Can you work these out from the model? Positions are in its coordinate system, mm. Face numbers are marked on the shaded views. A direction names the side the tool comes from. Give positions to 0.01 mm unless a question says otherwise; leave off trailing zeros. Order: outer loops, then holes, each group sorted by start corner. A loop starts at its lowest first (then second) coordinate and runs counter-clockwise, first axis right, second up. Notation, with made-up numbers: M 79,16 L 89,16 A31 ccw 89,52 Z; hole C 40.5,-15 d11. An arc over 180 degrees is marked long. Use one line per item in the form item = value. Start each with the question number.
1. We'd pull the mould along X, two halves only. Please class the marked faces 1, 2, 3 and 4: +X half, -X half, draft (parallel to the pull), parting line (faces both ways), or undercut.
2. I want a section at A-A, the plane z = -29.1. List the corners of the cut face in (x, y) for me, and give its area (3 significant figures).
3. I want a section at C-C, the plane z = -41.5. List the corners of the cut face in (x, y) for me.
4. Will this pin go through, and if not, where does the flat tip stop? P1, Ø11.5, axis at y = 397.93, z = -29.1, coming from the -X side.
5. I need wall thicknesses on L1, parallel to Y at x = -13.5, z = -29.1; L2, parallel to Z at x = 6, y = 488; L3, parallel to X at y = 475, z = -33.5. Which ranges of each line are inside material? Lowest first, please.
6. For the marked faces 5 and 6, which set-ups out of +Z, -Z, +X, -X, +Y, -Y let a thin tool reach every point of the face, with its end or its side?
7. I want a section at B-B, the plane x = -3.75. List the corners of the cut face in (y, z) for me, and give its area (3 significant figures).
8. I want a section at D-D, the plane y = 459. List the corners of the cut face in (x, z) for me, and give its area (3 significant figures).
```python
from build123d import *

# Parameters (mm, degrees)
CROQUIS1_W                        = 30
CROQUIS1_H                        = 119.965463257
SALIENTE_EXTRUIR1_DEPTH           = 30
CROQUIS2_W                        = 24
CROQUIS2_H                        = 24
CORTAR_EXTRUIR1_DEPTH             = 120.965463257
DI_METRO_DE_TALADRO_9_0_9_1_D     = 9
DI_METRO_DE_TALADRO_9_0_9_1_DEPTH = 3
DI_METRO_DE_TALADRO_9_0_9_2_D     = 9
DI_METRO_DE_TALADRO_9_0_9_2_DEPTH = 30
REDONDEO1_R                       = 3


with BuildPart() as part:
    # Croquis1 → Saliente-Extruir1 (new body)
    with BuildSketch(Plane.XY.offset(-20.120137415)):
        with Locations((0, 447.917268372)):
            Rectangle(CROQUIS1_W, CROQUIS1_H)
    extrude(amount=-SALIENTE_EXTRUIR1_DEPTH)

    # Croquis2 → Cortar-Extruir1 (cut, through all)
    with BuildSketch(Plane(origin=(0, 507.9, 0), x_dir=(-1, 0, 0), z_dir=(0, 1, 0))):
        with Locations((0, -35.120137415)):
            Rectangle(CROQUIS2_W, CROQUIS2_H)
    extrude(amount=-CORTAR_EXTRUIR1_DEPTH, mode=Mode.SUBTRACT)

    # Diámetro de taladro Ø9.0 (9)1
    with Locations(Plane(origin=(-12, 0, 0), x_dir=(0, 0, -1), z_dir=(1, 0, 0))):
        with Locations((29.1, 397.9345), (29.1, 497.9345)):
            Hole(DI_METRO_DE_TALADRO_9_0_9_1_D / 2, depth=DI_METRO_DE_TALADRO_9_0_9_1_DEPTH)

    # Diámetro de taladro Ø9.0 (9)2
    with Locations(Plane(origin=(15, 0, 0), x_dir=(0, 0, -1), z_dir=(1, 0, 0))):
        with Locations((29.1, 497.9345), (29.1, 397.9345)):
            Hole(DI_METRO_DE_TALADRO_9_0_9_2_D / 2, depth=DI_METRO_DE_TALADRO_9_0_9_2_DEPTH)

    # Redondeo1
    redondeo1_edges = [part.edges().sort_by_distance(p)[0] for p in [
        (15, 447.917268372, -50.120137415),
        (-15, 447.917268372, -50.120137415),
        (15, 447.917268372, -20.120137415),
        (-15, 447.917268372, -20.120137415),
    ]]
    fillet(redondeo1_edges, radius=REDONDEO1_R)


solid = part.part
```
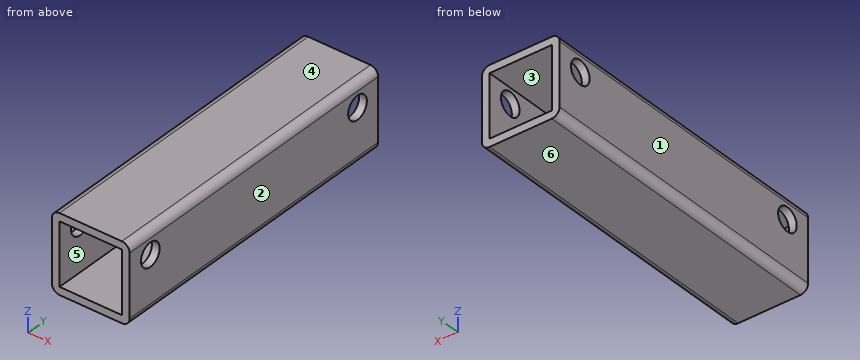
Check result:
q1.face_1 = -X half
q1.face_2 = +X half
q1.face_3 = undercut
q1.face_4 = draft
q2.outline = M -15,387.93 L -12,387.93 L -12,393.43 L -15,393.43 Z; M -15,402.43 L -12,402.43 L -12,493.43 L -15,493.43 Z; M -15,502.43 L -12,502.43 L -12,507.9 L -15,507.9 Z; M 12,387.93 L 15,387.93 L 15,393.43 L 12,393.43 Z; M 12,402.43 L 15,402.43 L 15,493.43 L 12,493.43 Z; M 12,502.43 L 15,502.43 L 15,507.9 L 12,507.9 Z
q2.area = 612 mm2
q3.outline = M -15,387.93 L -12,387.93 L -12,507.9 L -15,507.9 Z; M 12,387.93 L 15,387.93 L 15,507.9 L 12,507.9 Z
q4.P1 = -15
q5.L1 = 387.93 to 393.43, 402.43 to 493.43, 502.43 to 507.9
q5.L2 = -50.12 to -47.12, -23.12 to -20.12
q5.L3 = -15 to -12, 12 to 15
q6.face_5 = +Y, -Y
q6.face_6 = -Z, +X, -X, +Y, -Y
q7.outline = M 387.93,-50.12 L 507.9,-50.12 L 507.9,-47.12 L 387.93,-47.12 Z; M 387.93,-23.12 L 507.9,-23.12 L 507.9,-20.12 L 387.93,-20.12 Z
q7.area = 720 mm2
q8.outline = M -15,-47.12 A3 ccw -12,-50.12 L 12,-50.12 A3 ccw 15,-47.12 L 15,-23.12 A3 ccw 12,-20.12 L -12,-20.12 A3 ccw -15,-23.12 Z; hole M -12,-47.12 L 12,-47.12 L 12,-23.12 L -12,-23.12 Z
q8.area = 316 mm2
